Check sheet for the modelled part. Datum: model origin and axes. Units: mm. A direction names the side the tool comes from. Round coordinates to 2 decimals unless told otherwise and drop trailing zeros. Order: outer loops, then holes, each group sorted by start corner. A loop starts at its lowest first (then second) coordinate and runs counter-clockwise, first axis right, second up.
```python
from build123d import *

# Parameters (mm, degrees)
PAD_DEPTH     = 4
SKETCH001_W   = 2.5
SKETCH001_H   = 6
PAD001_DEPTH  = 30
SKETCH002_R   = 1.2
SKETCH002_R_2 = 1.6
POCKET_DEPTH  = 25.001


with BuildPart() as part:
    # Sketch → Pad (new body)
    with BuildSketch(Plane.XY):
        Polygon((-7.5, -20.000802), (-2.5, -20.000802), (-2.5, -16.000802), (2.5, -16.000802), (2.5, -20.000802), (7.5, -20.000802), (7.5, -16.000802), (12.5, -16.000802), (12.5, 23.999198), (-12.5, 23.999198), (-12.5, -16.000802), (-7.5, -16.000802), align=None)
    extrude(amount=PAD_DEPTH)

    # Sketch001 → Pad001 (new body)
    with BuildSketch(Plane.XY.offset(4)):
        with Locations((-11.25, -13.000802)):
            Rectangle(SKETCH001_W, SKETCH001_H)
        with Locations((-11.25, 20.999198)):
            Rectangle(SKETCH001_W, SKETCH001_H)
    extrude(amount=PAD001_DEPTH)

    # Sketch002 → Pocket (cut, through all)
    with BuildSketch(Plane(origin=(-12.5, 0, 0), x_dir=(0, -1, 0), z_dir=(-1, 0, 0))):
        with Locations((18.000802, 2)):
            Circle(SKETCH002_R)
        with Locations((13.000802, 27.5)):
            Circle(SKETCH002_R_2)
        with Locations((-20.999198, 27.5)):
            Circle(SKETCH002_R_2)
    extrude(amount=-POCKET_DEPTH, mode=Mode.SUBTRACT)


solid = part.part
```
Item 1: Access from +Z, -Z, +X, -X, +Y, -Y to the whole of each face (thin tool, end or side, straight path). Record for faces 1 (the flat face through (0, -16.001, 2)), 2 (the flat face through (-11, -10.001, 19)), 3 (the flat face through (-10, 21, 19)), 4 (the flat face through (7.5, -19, 3)), 5 (the flat face through (-11, -16.001, 17)).
Answer:
face 1: +Z, -Z, -Y
face 2: +Z, +X, -X
face 3: +Z, +X, +Y, -Y
face 4: +Z, -Z, +X, -Y
face 5: +Z, -Z, -X, -Y
Item 2: Sectioned sample at D-D (y = -8.5). Record the cut outline in (x, z).
Answer:
outline: (-12.5, 0) - (12.5, 0) - (12.5, 4) - (-12.5, 4) - close
Item 3: Sectioned sample at B-B (z = 17). Record the cut outline in (x, y).
Answer:
outline: (-12.5, -16) - (-10, -16) - (-10, -10) - (-12.5, -10) - close; (-12.5, 18) - (-10, 18) - (-10, 24) - (-12.5, 24) - close
Item 4: Go/stop test with flat-tipped pins: P1, Ø1.8, axis at y = 21, z = 18.5, coming from the +X side; P2, Ø3, axis at x = -11.5, z = 17, coming from the -Y side; P3, Ø3, axis at y = -18, z = 2, coming from the +X side. Record where each tip stops, or that it passes through.
Answer:
P1: stops at x = -10
P2: stops at y = -16
P3: stops at x = 7.5
Item 5: Scan lines: line 1 along Z through (x, y) = (9.25, 20.5); line 2 along X through (y, z) = (20, 17.5). Record each from-to range of solid material in increasing order.
Answer:
line 1: z = 0 to 4
line 2: x = -12.5 to -10
Item 6: Sectioned sample at C-C (z = 27.5). Record the cut outline in (x, y), and give its area (3 significant figures).
Answer:
outline: (-12.5, -16) - (-10, -16) - (-10, -14.6) - (-12.5, -14.6) - close; (-12.5, -11.4) - (-10, -11.4) - (-10, -10) - (-12.5, -10) - close; (-12.5, 18) - (-10, 18) - (-10, 19.4) - (-12.5, 19.4) - close; (-12.5, 22.6) - (-10, 22.6) - (-10, 24) - (-12.5, 24) - close
area: 14.0 mm2
Item 7: Release check for a two-part mould opening along Y. For faces 6 (the flat face through (-7.5, -19, 3)), 7 (the flat face through (10, -16.001, 2)), 8 (the flat face through (-11, 17.999, 19)), 9 (the cylindrical face through (-11.268, -12.793, 29.086)) record: released by +Y, released by -Y, zero draft, split by the parting line, or undercut.
Answer:
face 6: zero draft
face 7: released by -Y
face 8: undercut
face 9: undercut
Item 8: Sectioned sample at A-A (z = 2). Record the cut outline in (x, y), and give its area (3 significant figures).
Answer:
outline: (-12.5, -16) - (-7.5, -16) - (-7.5, -16.8) - (-2.5, -16.8) - (-2.5, -16) - (2.5, -16) - (2.5, -16.8) - (7.5, -16.8) - (7.5, -16) - (12.5, -16) - (12.5, 24) - (-12.5, 24) - close; (-7.5, -20) - (-2.5, -20) - (-2.5, -19.2) - (-7.5, -19.2) - close; (2.5, -20) - (7.5, -20) - (7.5, -19.2) - (2.5, -19.2) - close
area: 1,020 mm2
